Read the model definition and answer for the solid it produces. Units are mm, in the model's axes. A direction names the side the tool comes from. Coordinates: 2 decimals unless noted, no trailing zeros. Loops run counter-clockwise (first coordinate to the right, second up) from the corner with the lowest first, then second, coordinate; pieces in that order, holes last. Notation, with made-up numbers: M 15.5,85.5 L 36.5,85.5 A14 ccw 36.5,97.5 Z; hole C 1,27 d7. An arc over 180 degrees is marked long. One line per item, written item: value. Start each with the question number.
1. The part is cut by section C-C (z = -2). State how many separate pieces and enclosed holes the cut face has, then the cut area to 3 significant figures.
2. The part is cut by section A-A (y = 3.5). Write down the section's boundary in (x, z), then the cut area to 3 significant figures.
3. The part is cut by section B-B (x = 23.5). Write down the section's boundary in (y, z), then the cut area to 3 significant figures.
4. The part is cut by section D-D (y = 21). Write down the section's boundary in (x, z).
5. Consider probe 1 along X at (y, z) = (18.5, 2); probe 2 along Y at (x, z) = (-32.5, -0.1); probe 3 along X at (y, z) = (37.5, 0). Determine where each line is inside the solid, lowest interval first.
6. Flat-ended cylindrical pins translate along their axes: pin 1 (1.5 mm diameter, centred on x = -2.5, z = 0, fed in from -Y); pin 2 (2.5 mm diameter, centred on y = 2.5, z = 1, fed in from -X). Find the tip coordinate at first contact, or state that the pin passes through.
7. For faces 1 (the face through (-30, 6, 0)), 2 (the face through (16.28, 34.93, 0.27)), 3 (the face through (8, 30, 0)), determine the directions among +Z, -Z, +X, -X, +Y, -Y from which every point of the face is accessible in a straight line to the end or side of a thin tool.
8. Determine the mould class of faces 4 (the face through (-30, 34, 0)), 5 (the face through (-23.72, 34.85, 0.27)), 6 (the face through (-36.07, 7.5, -0.04)) for opening direction X: +X half, -X half, draft (parallel to the pull), parting line (faces both ways), or undercut.
```python
from build123d import *

# Parameters (mm, degrees)
SKETCH1_W           = 55
SKETCH1_H           = 6
BOSS_EXTRUDE1_DEPTH = 40
M3_TAPPED_HOLE1_D   = 2.5
CUT_EXTRUDE1_DEPTH  = 40
CHAMFER1_SIZE       = 1
SKETCH9_R           = 1.75
BOSS_EXTRUDE4_DEPTH = 6


with BuildPart() as part:
    # Sketch1 → Boss-Extrude1 (new body)
    with BuildSketch(Plane(origin=(0, 0, 0), x_dir=(1, 0, 0), z_dir=(0, 1, 0))):
        Rectangle(SKETCH1_W, SKETCH1_H)
    extrude(amount=BOSS_EXTRUDE1_DEPTH)

    # M3 Tapped Hole1 (through all)
    with Locations(Plane(origin=(-22.5, 40, 0), x_dir=(0, 0, 1), z_dir=(0, 1, 0))):
        with Locations((0, 0), (0, 20), (0, 40)):
            Hole(M3_TAPPED_HOLE1_D / 2)

    # Sketch7 → Cut-Extrude1 (cut)
    with BuildSketch(Plane(origin=(0, 0, -3), x_dir=(-1, 0, 0), z_dir=(0, 0, -1))):
        with BuildLine():
            Line((27.5, 30), (22.5, 30))
            ThreePointArc((22.5, 30), (18.964466094, 28.535533906), (17.5, 25))
            Line((17.5, 25), (17.5, 15))
            ThreePointArc((17.5, 15), (18.964466094, 11.464466094), (22.5, 10))
            Line((22.5, 10), (27.5, 10))
            Line((27.5, 10), (27.5, 30))
        make_face()
        with BuildLine():
            Line((4.5, 30), (-20.5, 30))
            ThreePointArc((-20.5, 30), (-24.035533906, 28.535533906), (-25.5, 25))
            Line((-25.5, 25), (-25.5, 15))
            ThreePointArc((-25.5, 15), (-24.035533906, 11.464466094), (-20.5, 10))
            Line((-20.5, 10), (4.5, 10))
            ThreePointArc((4.5, 10), (8.035533906, 11.464466094), (9.5, 15))
            Line((9.5, 15), (9.5, 25))
            ThreePointArc((9.5, 25), (8.035533906, 28.535533906), (4.5, 30))
        make_face()
    extrude(amount=-CUT_EXTRUDE1_DEPTH, mode=Mode.SUBTRACT)

    # Chamfer1
    chamfer1_edges = [part.edges().sort_by_distance(p)[0] for p in [
        (-27.5, 40, 0),
        (27.5, 40, 0),
        (-27.5, 0, 0),
        (27.5, 0, 0),
    ]]
    chamfer(chamfer1_edges, length=CHAMFER1_SIZE)

    # Sketch9 → Boss-Extrude4 (add)
    with BuildSketch(Plane(origin=(0, 0, -3), x_dir=(-1, 0, 0), z_dir=(0, 0, -1))):
        with BuildLine():
            Line((27.5, 34), (32.5, 34))
            ThreePointArc((32.5, 34), (36.035533906, 32.535533906), (37.5, 29))
            Line((37.5, 29), (37.5, 11))
            ThreePointArc((37.5, 11), (36.035533906, 7.464466094), (32.5, 6))
            Line((32.5, 6), (27.5, 6))
            Line((27.5, 6), (27.5, 34))
        make_face()
        with Locations((32.5, 27)):
            Circle(SKETCH9_R, mode=Mode.SUBTRACT)
        with Locations((32.5, 13)):
            Circle(SKETCH9_R, mode=Mode.SUBTRACT)
    extrude(amount=-BOSS_EXTRUDE4_DEPTH)


solid = part.part
```
Answer block:
1. separate pieces: 1
1. enclosed holes: 4
1. area: 1,580 mm2
2. outline: M -27.5,-3 L 27.5,-3 L 27.5,3 L -27.5,3 Z; hole C -22.5,0 d2.5; hole C -2.5,0 d2.5; hole C 17.5,0 d2.5
2. area: 315 mm2
3. outline: M 0,-3 L 11,-3 L 11,3 L 0,3 Z; M 29,-3 L 40,-3 L 40,3 L 29,3 Z
3. area: 132 mm2
4. outline: M -37.5,-3 L -27.5,-3 L -27.5,3 L -37.5,3 Z; M -17.5,-3 L -9.5,-3 L -9.5,3 L -17.5,3 Z; M 25.5,-3 L 27.5,-3 L 27.5,3 L 25.5,3 Z
5. probe 1: x = -37.5 to -27.5, -17.5 to -9.5, 25.5 to 27.5
5. probe 2: y = 6 to 11.25, 14.75 to 25.25, 28.75 to 34
5. probe 3: x = -27.5 to -23.75, -21.25 to -3.75, -1.25 to 16.25, 18.75 to 27.5
6. pin 1: passes through
6. pin 2: stops at x = -27.5
7. face 1: +Z, -Z, -X, -Y
7. face 2: +Y, -Y
7. face 3: +Z, -Z
8. face 4: draft
8. face 5: undercut
8. face 6: -X half
